Read the model definition and answer for the solid it produces. Units are mm, in the model's axes. A direction names the side the tool comes from. Coordinates: 2 decimals unless noted, no trailing zeros. Loops run counter-clockwise (first coordinate to the right, second up) from the corner with the lowest first, then second, coordinate; pieces in that order, holes last. Notation, with made-up numbers: (33, 78) -> (41, 78) arc R20 ccw to (41, 114) -> close; hole circle Ø5 at (46, 64). An arc over 180 degrees is marked (long way). Answer as a JSON object with one key per item and string values. Group by question number.
Q1. The part is cut by section C-C on y = 10. Write down the section's boundary in (x, z), and give its area (3 significant figures).
Q2. Straight lines are drawn through the part: line 1 along Z through (x, y) = (15, 1.1); line 2 along Z through (x, y) = (11.5, 1.5); line 3 along Z through (x, y) = (20, 0.85) (3 decimals). For each, find the intervals that lie inside material, in ascending order. Write a range as [from, to].
Q3. The part is cut by section A-A on z = 150. Write down the section's boundary in (x, y).
Q4. The part is cut by section D-D on z = 43.5. Write down the section's boundary in (x, y), and give its area (3 significant figures).
Q5. Determine the mould class of faces 1 (the cylindrical face through (19.153, 0.986, 242.015)), 2 (the flat face through (11, 1, 300)), 3 (the flat face through (2, 9, 148)), 4 (the flat face through (11, 1, 0)) for opening direction Z: released by +Z, released by -Z, zero draft, split by the parting line, or undercut.
Q6. The part is cut by section B-B on z = 191.5. Write down the section's boundary in (x, y).
Q7. Each of these flat-tipped pins is pushed along its axis until it touches: P1, Ø4, axis at x = 23, z = 240.5, coming from the +Y side; P2, Ø2, axis at y = 6.5, z = 197.5, coming from the +X side; P3, Ø3.5, axis at x = 10, z = 10, coming from the +Y side. Where does it stop, or does it pass through?
Q8. For faces 5 (the flat face through (0, 7, 148)), 6 (the flat face through (25, 2, 148)), determine the directions among +Z, -Z, +X, -X, +Y, -Y from which every point of the face is accessible in a straight line to the end or side of a thin tool.
from build123d import *

# Parameters (mm, degrees)
BOSS_EXTRUDE1_DEPTH = 300
SKETCH2_R           = 8
SKETCH2_R_2         = 1.977693409
CUT_EXTRUDE1_DEPTH  = 10
SKETCH3_W           = 300
SKETCH3_H           = 10
CUT_EXTRUDE2_DEPTH  = 10
SKETCH6_R           = 9
CUT_EXTRUDE5_DEPTH  = 5


with BuildPart() as part:
    # Sketch1 → Boss-Extrude1 (new body)
    with BuildSketch(Plane.XY):
        Polygon((0, 0), (0, 25), (2, 25), (2, 2), (30, 2), (30, 0), align=None)
    extrude(amount=BOSS_EXTRUDE1_DEPTH)

    # Sketch2 → Cut-Extrude1 (cut)
    with BuildSketch(Plane(origin=(0, 2, 0), x_dir=(1, 0, 0), z_dir=(0, 1, 0))):
        with Locations(Location((15, -150, 0), (0, 0, 180))):
            Circle(SKETCH2_R)
        with Locations(Location((10, -10, 0), (0, 0, 180))):
            Circle(SKETCH2_R_2)
        with Locations(Location((20, -20, 0), (0, 0, 180))):
            Circle(SKETCH2_R_2)
        with Locations(Location((10, -290, 0), (0, 0, 180))):
            Circle(SKETCH2_R_2)
        with Locations(Location((20, -280, 0), (0, 0, 180))):
            Circle(SKETCH2_R_2)
    extrude(amount=-CUT_EXTRUDE1_DEPTH, mode=Mode.SUBTRACT)

    # Sketch3 → Cut-Extrude2 (cut)
    with BuildSketch(Plane(origin=(2, 0, 0), x_dir=(0, 0, -1), z_dir=(1, 0, 0))):
        with Locations((-150, 20)):
            Rectangle(SKETCH3_W, SKETCH3_H)
    extrude(amount=-CUT_EXTRUDE2_DEPTH, mode=Mode.SUBTRACT)

    # Sketch6 → Cut-Extrude5 (cut)
    with BuildSketch(Plane.XZ):
        with Locations((15, 250)):
            Circle(SKETCH6_R)
        with Locations((15, 50)):
            Circle(SKETCH6_R)
        with Locations((-238, 50)):
            Circle(SKETCH6_R)
        with Locations((-238, 250)):
            Circle(SKETCH6_R)
    extrude(amount=-CUT_EXTRUDE5_DEPTH, mode=Mode.SUBTRACT)


solid = part.part
Final values:
{
 "1": {"outline": "(0, 0) -> (2, 0) -> (2, 300) -> (0, 300) -> close", "area": "600 mm2"},
 "2": {"line 1": "z = [0, 41], [59, 142], [158, 241], [259, 300]", "line 2": "z = [0, 8.71], [11.29, 41.71], [58.29, 142.81], [157.19, 241.71], [258.29, 288.71], [291.29, 300]", "line 3": "z = [0, 18.022], [21.978, 42.517], [57.483, 143.755], [156.245, 242.517], [257.483, 278.022], [281.978, 300]"},
 "3": {"outline": "(0, 0) -> (7, 0) -> (7, 2) -> (2, 2) -> (2, 15) -> (0, 15) -> close; (23, 0) -> (30, 0) -> (30, 2) -> (23, 2) -> close"},
 "4": {"outline": "(0, 0) -> (8.78, 0) -> (8.78, 2) -> (2, 2) -> (2, 15) -> (0, 15) -> close; (21.22, 0) -> (30, 0) -> (30, 2) -> (21.22, 2) -> close", "area": "61.1 mm2"},
 "5": {"face 1": "undercut", "face 2": "released by +Z", "face 3": "zero draft", "face 4": "released by -Z"},
 "6": {"outline": "(0, 0) -> (30, 0) -> (30, 2) -> (2, 2) -> (2, 15) -> (0, 15) -> close"},
 "7": {"P1": "stops at y = 2", "P2": "stops at x = 2", "P3": "passes through"},
 "8": {"face 5": "+Z, -Z, -X, +Y, -Y", "face 6": "+Z, -Z, +X, +Y"}
}
